Can you work these out from the drawing? Everything is in mm from the part's minimum corner. A direction names the side the tool comes from. Round coordinates to 2 decimals unless told otherwise and drop trailing zeros. Order: outer loops, then holes, each group sorted by start corner. A loop starts at its lowest first (then second) coordinate and runs counter-clockwise, first axis right, second up. Notation, with made-up numbers: (48, 47) -> (66, 47) arc R23 ccw to (66, 82) -> close; hole circle Ø11 at (3.5, 35.25). An arc over 180 degrees is marked (long way). One line per item, written item: value.
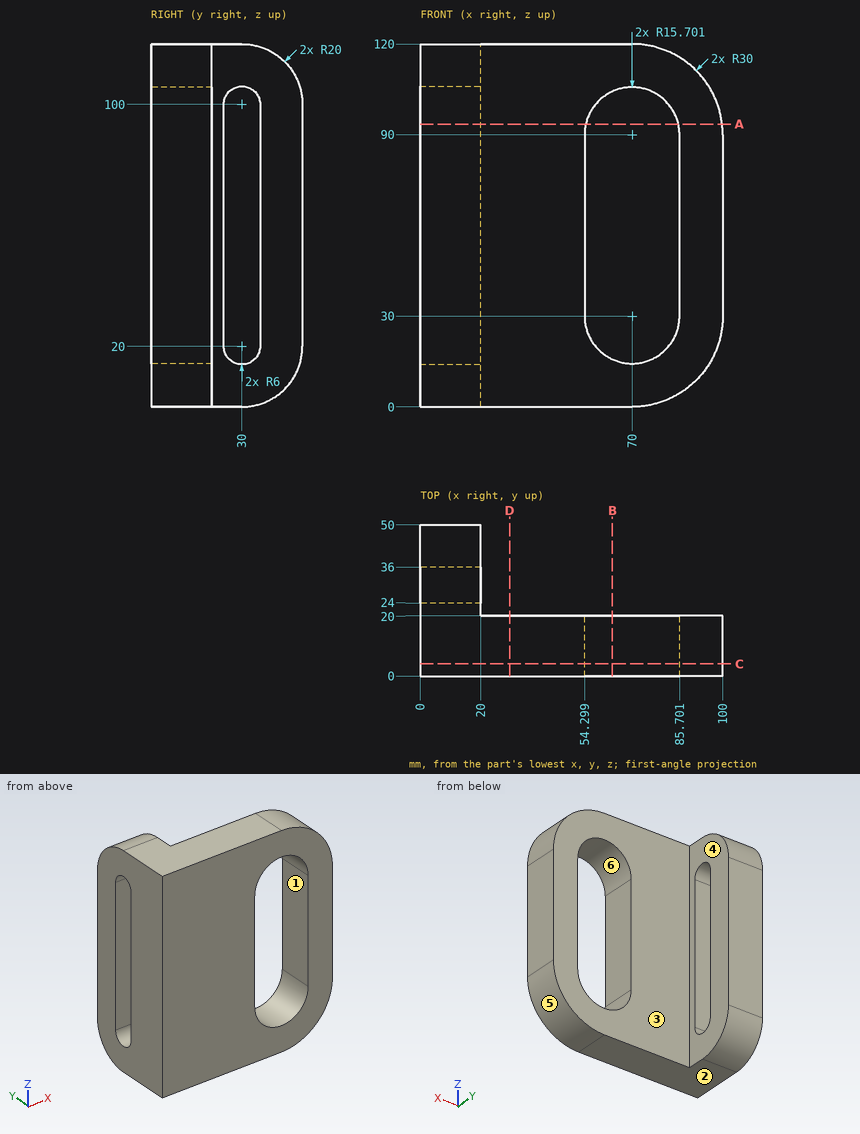
Q1. Please list where these lines run through material, in increasing order: line 1 along X through (y, z) = (7, 29.5); line 2 along Y through (x, z) = (6, 56); line 3 along Y through (x, z) = (85, 98.5).
Answers below:
line 1: 0 to 54.31, 85.69 to 100
line 2: 0 to 24, 36 to 50
line 3: 0 to 20
Q2. Will these pins go through, and if not, where does the flat tip stop? pin 1 Ø4 at (y, z) = (23, 81.5) entering from +X; pin 2 Ø5 at (y, z) = (11, 15) entering from +X.
Answers below:
pin 1: x = 20
pin 2: x = 97.27
Q3. We'd pull the mould along Z, two halves only. Please class the marked faces 1, 2 and 3: released by +Z, released by -Z, zero draft, split by the parting line, or undercut.
Answers below:
face 1: undercut
face 2: released by -Z
face 3: zero draft
Q4. I want a section at D-D on x = 29.5. List the corners of the cut face in (y, z) for me.
Answers below:
outline: (0, 0) -> (20, 0) -> (20, 120) -> (0, 120) -> close
Q5. I want a section at C-C on y = 4. List the corners of the cut face in (x, z) for me.
Answers below:
outline: (0, 0) -> (70, 0) arc R30 ccw to (100, 30) -> (100, 90) arc R30 ccw to (70, 120) -> (0, 120) -> close; hole (54.3, 30) arc R15.7 ccw to (85.7, 30) -> (85.7, 90) arc R15.7 ccw to (54.3, 90) -> close
Q6. I want a section at A-A on z = 93.5. List the corners of the cut face in (x, y) for me (3 decimals), plus the area to 3 significant figures.
Answers below:
outline: (0, 0) -> (54.694, 0) -> (54.694, 20) -> (20, 20) -> (20, 24) -> (0, 24) -> close; (0, 36) -> (20, 36) -> (20, 50) -> (0, 50) -> close; (85.306, 0) -> (99.795, 0) -> (99.795, 20) -> (85.306, 20) -> close
area: 1,740 mm^2
Q7. On a 3-axis mill with a long thin cutter (end or side, diameter ignored), from which of +Z, -Z, +X, -X, +Y, -Y can I reach the whole of each face in a straight line? I mean the marked faces 4, 5 and 6. Say none if no direction works.
Answers below:
face 4: +Z, -Z, +X, +Y
face 5: -Z, +X, +Y, -Y
face 6: +Y, -Y
Q8. I want a section at B-B on x = 63.5. List the corners of the cut face in (y, z) for me, plus the area to 3 significant figures.
Answers below:
outline: (0, 0) -> (20, 0) -> (20, 15.71) -> (0, 15.71) -> close; (0, 104.29) -> (20, 104.29) -> (20, 120) -> (0, 120) -> close
area: 628 mm^2
